```python
from build123d import *

# Parameters (mm, degrees)
BOSS_EXTRUDE1_DEPTH     = 3
CUT_EXTRUDE1_DEPTH      = 1894.152557487
CUT_EXTRUDE1_DEPTH_BACK = 1894.152557487
SKETCH3_R               = 2.75


with BuildPart() as part:
    # Sketch1 → Boss-Extrude1 (new body)
    with BuildSketch(Plane(origin=(661.48611704, 211.228421756, 131.566142626), x_dir=(0.17733557040624817, 0.05662751143705051, -0.9825199338523047), z_dir=(0.9359591821601212, 0.2988742708017776, 0.1861574053935612))):
        Polygon((-1711.561008488, 536.583768948), (-1818.35898353, 342.579279309), (-1328.661052703, 313.46937198), (-1355.956557086, 515.444997525), align=None)
    extrude(amount=BOSS_EXTRUDE1_DEPTH)

    # Sketch3 → Cut-Extrude1 (cut, two sides: drawn at the far end of the back side and taken through both)
    with BuildSketch(Plane(origin=(661.48611704, 211.228421756, 131.566142626), x_dir=(0.17733557040624817, 0.05662751143705051, -0.9825199338523047), z_dir=(0.9359591821601212, 0.2988742708017776, 0.1861574053935612)).offset(-CUT_EXTRUDE1_DEPTH_BACK)):
        with Locations(Location((-1729.277570286, 448.219803938, 0), (0, 0, 90))):
            Circle(SKETCH3_R)
        with Locations(Location((-1762.245431769, 388.21613765, 0), (0, 0, 90))):
            Circle(SKETCH3_R)
        with Locations(Location((-1365.280056563, 364.618681835, 0), (0, 0, 90))):
            Circle(SKETCH3_R)
        with Locations(Location((-1373.721769773, 427.083924548, 0), (0, 0, 90))):
            Circle(SKETCH3_R)
    extrude(amount=CUT_EXTRUDE1_DEPTH + CUT_EXTRUDE1_DEPTH_BACK, mode=Mode.SUBTRACT)


solid = part.part
```
CAD build for the part. Positions are in the model's coordinates, mm. Round coordinates to 2 decimals unless told otherwise and drop trailing zeros. Order: outer loops, then holes, each group sorted by start corner. A loop starts at its lowest first (then second) coordinate and runs counter-clockwise, first axis right, second up. Notation, with made-up numbers: (-38, 44.25) - (-14, 44.25) arc R13 cw to (-14, 59.25) - close; hole circle Ø8 at (75, 78.5). An arc over 180 degrees is marked (long way). Use CSV: the item, a comma, the result in double quotes. Start each with the question number.
1) Pin check, flat tips, straight feed: pin 1 Ø1.5 at (y, z) = (585, 1736) entering from +X; pin 2 Ø1 at (y, z) = (515.5, 1571) entering from -X; pin 3 Ø8 at (x, z) = (264, 1495) entering from +Y; pin 4 Ø1 at (x, y) = (316.5, 489) entering from -Z. Stop position of each tip, or through.
2) Wall check: L1, parallel to X at y = 562, z = 1516; L2, parallel to X at y = 611, z = 1791.5. Give the ranges that are in metal, low to high. Write a range as [from, to].
3) Saw through at A-A (x = 208). List the corners of the cut face in (y, z).
4) Saw through at B-B (z = 1616). List the corners of the cut face in (x, y).
Values follow:
1,pin 1,"stops at x = 226.51"
1,pin 2,"stops at x = 277.84"
1,pin 3,"stops at y = 626.36"
1,pin 4,"passes through"
2,L1,"x = [274.12, 277.32]"
2,L2,"x = [203.68, 206.88]"
3,outline,"(562.32, 1847.92) - (625.46, 1746.55) - (626.36, 1761.22) - (576.59, 1841.13) - close"
4,outline,"(233.97, 625.46) - (294.91, 434.6) - (297.83, 435.5) - (236.88, 626.36) - close"
